```python
from build123d import *

# Parameters (mm, degrees)
SKETCH_1_W          = 50
SKETCH_1_H          = 20
EXTRUDE_1_DEPTH     = 5
SKETCH_2_W          = 34
SKETCH_2_H          = 20
EXTRUDE_2_DEPTH     = 5
SKETCH_3_R          = 1.6
CUT_EXTRUDE_1_DEPTH = 5


with BuildPart() as part:
    # 草图1 → 凸台-拉伸1 (new body)
    with BuildSketch(Plane.XY):
        with Locations((15.734265734, 15.34965035)):
            Rectangle(SKETCH_1_W, SKETCH_1_H)
    extrude(amount=EXTRUDE_1_DEPTH)

    # 草图2 → 凸台-拉伸2 (add)
    with BuildSketch(Plane.XY.offset(5)):
        with Locations((15.734265734, 15.34965035)):
            Rectangle(SKETCH_2_W, SKETCH_2_H)
    extrude(amount=EXTRUDE_2_DEPTH)

    # 草图3 → 切除-拉伸1 (cut)
    with BuildSketch(Plane.XY.offset(5)):
        with Locations((-5.265734266, 15.34965035)):
            Circle(SKETCH_3_R)
        with Locations((36.734265734, 15.34965035)):
            Circle(SKETCH_3_R)
    extrude(amount=-CUT_EXTRUDE_1_DEPTH, mode=Mode.SUBTRACT)


solid = part.part
```
The listing builds one solid part. Answer for the finished solid, in the listing's coordinates (mm). A direction names the side the tool comes from. Give positions to 0.01 mm unless a question says otherwise; leave off trailing zeros. Loops run counter-clockwise (first coordinate to the right, second up) from the corner with the lowest first, then second, coordinate; pieces in that order, holes last. Notation, with made-up numbers: (-12, 65) - (38, 65) arc R25 ccw to (38, 92) - close; hole circle Ø6 at (74, -33). An arc over 180 degrees is marked (long way). Return JSON: item names as keys, results as strings. Group by question number.
1. Straight lines are drawn through the part: line 1 (X direction, y = 15.25, z = 1.25); line 2 (Z direction, x = 38.5, y = 8.5); line 3 (X direction, y = 20, z = 9). For each, find the intervals that lie inside material, in ascending order. Write a range as [from, to].
2. Find section C-C (z = 4.25). Write down the section's boundary in (x, y).
3. Find section A-A (x = -5). Write down the section's boundary in (y, z).
4. Find section D-D (z = 7). Write down the section's boundary in (x, y).
5. Find section B-B (y = 7.75). Write down the section's boundary in (x, z), then the cut area to 3 significant figures.
6. Which of the six approach directions +Z, -Z, +X, -X, +Y, -Y give full straight-line access (tool end or side, diameter ignored) to faces 1 (the flat face through (-7, 15, 5)), 2 (the flat face through (15, 5.35, 5)), 3 (the flat face through (32.734, 15, 7))?
7. Given pin 1 Ø5 at (x, y) = (21.5, 21) entering from -Z; pin 2 Ø6.5 at (x, y) = (-6.5, 11.5) entering from +Z; pin 3 Ø1.5 at (y, z) = (15.5, 7) entering from +X; pin 4 Ø5.5 at (y, z) = (14, 8.5) entering from -X, each flat-ended and moving along its own axis, determine where each tip first touches the part or whether it passes through.
8. Determine the mould class of faces 4 (the cylindrical face through (35.136, 15.42, 2.535)), 5 (the flat face through (-9.266, 15, 2)), 6 (the flat face through (15, 25.35, 5)) for opening direction Y: pulls with the +Y half, pulls with the -Y half, needs draft (parallel to the pull), parting line crosses it, or undercut.
Verdict:
{
 "1": {"line 1": "x = [-9.27, -6.86], [-3.67, 35.14], [38.33, 40.73]", "line 2": "z = [0, 5]", "line 3": "x = [-1.27, 32.73]"},
 "2": {"outline": "(-9.27, 5.35) - (40.73, 5.35) - (40.73, 25.35) - (-9.27, 25.35) - close; hole circle Ø3.2 at (-5.27, 15.35); hole circle Ø3.2 at (36.73, 15.35)"},
 "3": {"outline": "(5.35, 0) - (13.77, 0) - (13.77, 5) - (5.35, 5) - close; (16.93, 0) - (25.35, 0) - (25.35, 5) - (16.93, 5) - close"},
 "4": {"outline": "(-1.27, 5.35) - (32.73, 5.35) - (32.73, 25.35) - (-1.27, 25.35) - close"},
 "5": {"outline": "(-9.27, 0) - (40.73, 0) - (40.73, 5) - (32.73, 5) - (32.73, 10) - (-1.27, 10) - (-1.27, 5) - (-9.27, 5) - close", "area": "420 mm^2"},
 "6": {"face 1": "+Z, -X, +Y, -Y", "face 2": "+Z, -Z, +X, -X, -Y", "face 3": "+Z, +X, +Y, -Y"},
 "7": {"pin 1": "stops at z = 0", "pin 2": "stops at z = 5", "pin 3": "stops at x = 32.73", "pin 4": "stops at x = -1.27"},
 "8": {"face 4": "undercut", "face 5": "needs draft", "face 6": "pulls with the +Y half"}
}
